CAD build for the part. Positions are in the model's coordinates, mm. Give positions to 0.01 mm unless a question says otherwise; leave off trailing zeros. Order: outer loops, then holes, each group sorted by start corner. A loop starts at its lowest first (then second) coordinate and runs counter-clockwise, first axis right, second up. Notation, with made-up numbers: M 52,71 L 75,71 A10 ccw 75,76 Z; hole C 10.25,56.25 d2. An arc over 180 degrees is marked long. Put each result on its own line as item: value. Start each with the question number.
1) Two-plate mould, pull along Y, no slides. Class faces 1 (the face through (41.34, -22.89, 0.04)), 2 (the face through (41.34, 27.11, 0.04)), 3 (the face through (-1, 1, -2.5)), 4 (the face through (1, 37.5, 0)): released by +Y, released by -Y, zero draft, split by the parting line, or undercut.
2) Drill centre lines: line 1 (Y direction, x = -40, z = -0.8); line 2 (Y direction, x = -38.5, z = -1.85); line 3 (X direction, y = -28, z = -1.1). Where is each one in solid material? Low to high. Write a range as [from, to].
3) Pin check, flat tip, straight feed: pin 1 (4 mm diameter, centred on x = 40, y = -25, fed in from +Z). Stop position of the tip, or through.
4) Cut at A-A (y = -25). Write the cut outline in (x, z), and give its area (3 significant figures).
5) Cut at B-B (z = 0.9). Write the cut outline in (x, y).
```python
from build123d import *

# Parameters (mm, degrees)
SKETCH1_R           = 12.5
BOSS_EXTRUDE1_DEPTH = 2.5
SKETCH2_R           = 2.5
CUT_EXTRUDE1_DEPTH  = 63.69968102
SKETCH5_R           = 12.5
BOSS_EXTRUDE2_DEPTH = 2.5


with BuildPart() as part:
    # Sketch1 → Boss-Extrude1 (new, symmetric)
    with BuildSketch(Plane.XY):
        with BuildLine():
            Line((-40, -37.5), (40, -37.5))
            ThreePointArc((40, -37.5), (47.071067812, -34.571067812), (50, -27.5))
            Line((50, -27.5), (50, 27.5))
            ThreePointArc((50, 27.5), (47.071067812, 34.571067812), (40, 37.5))
            Line((40, 37.5), (-40, 37.5))
            ThreePointArc((-40, 37.5), (-47.071067812, 34.571067812), (-50, 27.5))
            Line((-50, 27.5), (-50, -27.5))
            ThreePointArc((-50, -27.5), (-47.071067812, -34.571067812), (-40, -37.5))
        make_face()
        Circle(SKETCH1_R, mode=Mode.SUBTRACT)
    extrude(amount=BOSS_EXTRUDE1_DEPTH, both=True)

    # Sketch2 → Cut-Extrude1 (cut, through all)
    with BuildSketch(Plane.XY.offset(2.5)):
        with Locations((40, 25)):
            Circle(SKETCH2_R)
        with Locations((-40, 25)):
            Circle(SKETCH2_R)
        with Locations((-40, -25)):
            Circle(SKETCH2_R)
        with Locations((40, -25)):
            Circle(SKETCH2_R)
    extrude(amount=-CUT_EXTRUDE1_DEPTH, mode=Mode.SUBTRACT)

    # Sketch5 → Boss-Extrude2 (add, symmetric)
    with BuildSketch(Plane.XY):
        Circle(SKETCH5_R)
    extrude(amount=BOSS_EXTRUDE2_DEPTH, both=True)


solid = part.part
```
Solution:
1. face 1: undercut
1. face 2: undercut
1. face 3: zero draft
1. face 4: released by +Y
2. line 1: [-37.5, -27.5], [-22.5, 22.5], [27.5, 37.5]
2. line 2: [-37.5, -27], [-23, 23], [27, 37.5]
2. line 3: [-49.99, 49.99]
3. pin 1: through
4. outline: M -50,-2.5 L -42.5,-2.5 L -42.5,2.5 L -50,2.5 Z; M -37.5,-2.5 L 37.5,-2.5 L 37.5,2.5 L -37.5,2.5 Z; M 42.5,-2.5 L 50,-2.5 L 50,2.5 L 42.5,2.5 Z
4. area: 450 mm²
5. outline: M -50,-27.5 A10 ccw -40,-37.5 L 40,-37.5 A10 ccw 50,-27.5 L 50,27.5 A10 ccw 40,37.5 L -40,37.5 A10 ccw -50,27.5 Z; hole C -40,-25 d5; hole C -40,25 d5; hole C 40,-25 d5; hole C 40,25 d5
